```python
from build123d import *

# Parameters (mm, degrees)
ESQUISSE1_W         = 40.75
ESQUISSE1_H         = 20.6
EXTRUSION1_DEPTH    = 9.26
ESQUISSE2_R         = 1.25
EXTRUSION2_DEPTH    = 47.590450738
ESQUISSE4_OUTSIDE_W = 52.068
ESQUISSE4_OUTSIDE_H = 31.918
EXTRUSION5_DEPTH    = 47.590450738
EXTRUSION4_START    = -1.3
EXTRUSION4_DEPTH    = 1.3
EXTRUSION9_DEPTH    = 7.8
EXTRUSION10_REACH   = 48.59
ESQUISSE7_W         = 4
ESQUISSE7_H         = 8.124058542
ESQUISSE8_R         = 2.5
EXTRUSION11_DEPTH   = 4
CONG_1_R            = 5
ESQUISSE9_R         = 2.1
EXTRUSION12_DEPTH   = 1.3


with BuildPart() as part:
    # Esquisse1 → Extrusion1 (new body)
    with BuildSketch(Plane.XY):
        with Locations((-20.375, 10.3)):
            Rectangle(ESQUISSE1_W, ESQUISSE1_H)
    extrude(amount=EXTRUSION1_DEPTH)

    # Esquisse2 → Extrusion2 (cut, through all)
    with BuildSketch(Plane.XY.offset(9.26)):
        with Locations((-38, 17.85)):
            Circle(ESQUISSE2_R)
        with Locations(Location((-38, 2.75, 0), (0, 0, 180))):
            Circle(ESQUISSE2_R)
        with Locations((-2.75, 2.75)):
            Circle(ESQUISSE2_R)
        with Locations(Location((-2.75, 17.85, 0), (0, 0, 180))):
            Circle(ESQUISSE2_R)
    extrude(amount=-EXTRUSION2_DEPTH, mode=Mode.SUBTRACT)

    # Esquisse4 outside → Extrusion5 (cut, through all)
    with BuildSketch(Plane(origin=(0, 0, 0), x_dir=(-1, 0, 0), z_dir=(0, 0, -1))):
        with Locations((20.375, 10.3)):
            Rectangle(ESQUISSE4_OUTSIDE_W, ESQUISSE4_OUTSIDE_H)
        with BuildLine():
            Line((2.75, 20.6), (38, 20.6))
            ThreePointArc((38, 20.6), (39.944543648, 19.794543648), (40.75, 17.85))
            Line((40.75, 17.85), (40.75, 2.75))
            ThreePointArc((40.75, 2.75), (39.944543648, 0.805456352), (38, 0))
            Line((38, 0), (2.75, 0))
            ThreePointArc((2.75, 0), (0.805456352, 0.805456352), (0, 2.75))
            Line((0, 2.75), (0, 17.85))
            ThreePointArc((0, 17.85), (0.805456352, 19.794543648), (2.75, 20.6))
        make_face(mode=Mode.SUBTRACT)
    extrude(amount=-EXTRUSION5_DEPTH, mode=Mode.SUBTRACT)

    # Esquisse3 → Extrusion4 (cut)
    with BuildSketch(Plane.XY.offset(9.26).offset(EXTRUSION4_START)):
        with BuildLine():
            Line((-38, 20.6), (-2.75, 20.6))
            ThreePointArc((-2.75, 20.6), (-0.805456352, 19.794543648), (0, 17.85))
            Line((0, 17.85), (0, 2.75))
            ThreePointArc((0, 2.75), (-0.805456352, 0.805456352), (-2.75, 0))
            Line((-2.75, 0), (-38, 0))
            ThreePointArc((-38, 0), (-39.944543648, 0.805456352), (-40.75, 2.75))
            Line((-40.75, 2.75), (-40.75, 17.85))
            ThreePointArc((-40.75, 17.85), (-39.944543648, 19.794543648), (-38, 20.6))
        make_face()
        with BuildLine():
            Line((-38, 19.6), (-2.75, 19.6))
            ThreePointArc((-2.75, 19.6), (-1.512563133, 19.087436867), (-1, 17.85))
            Line((-1, 17.85), (-1, 2.75))
            ThreePointArc((-1, 2.75), (-1.512563133, 1.512563133), (-2.75, 1))
            Line((-2.75, 1), (-38, 1))
            ThreePointArc((-38, 1), (-39.237436867, 1.512563133), (-39.75, 2.75))
            Line((-39.75, 2.75), (-39.75, 17.85))
            ThreePointArc((-39.75, 17.85), (-39.237436867, 19.087436867), (-38, 19.6))
        make_face(mode=Mode.SUBTRACT)
    extrude(amount=EXTRUSION4_DEPTH, mode=Mode.SUBTRACT)

    # Esquisse6 → Extrusion9 (cut)
    with BuildSketch(Plane.XY.offset(9.26)):
        with BuildLine():
            Line((-36.650926244, 18.8), (-4.099073756, 18.8))
            ThreePointArc((-4.099073756, 18.8), (-3.916726189, 16.683273811), (-1.8, 16.500926244))
            Line((-1.8, 16.500926244), (-1.8, 4.099073756))
            ThreePointArc((-1.8, 4.099073756), (-3.916726189, 3.916726189), (-4.099073756, 1.8))
            Line((-4.099073756, 1.8), (-36.650926244, 1.8))
            ThreePointArc((-36.650926244, 1.8), (-36.833273811, 3.916726189), (-38.95, 4.099073756))
            Line((-38.95, 4.099073756), (-38.95, 16.500926244))
            ThreePointArc((-38.95, 16.500926244), (-36.833273811, 16.683273811), (-36.650926244, 18.8))
        make_face()
    extrude(amount=-EXTRUSION9_DEPTH, mode=Mode.SUBTRACT)

    # Extrusion10: up to this face of the body (flat: up to its plane)
    extrusion10_end = Plane(part.part.faces().sort_by_distance((-38.95, 10.3, 5.36))[0])
    # Esquisse7 → Extrusion10 (cut, up to the picked face)
    with BuildSketch(Plane.ZY.offset(40.75), mode=Mode.PRIVATE) as extrusion10_sk1:
        with Locations((7.26, 10.3)):
            Rectangle(ESQUISSE7_W, ESQUISSE7_H)
    extrusion10_tool1 = split(extrude(extrusion10_sk1.sketch, amount=-EXTRUSION10_REACH, mode=Mode.PRIVATE), bisect_by=extrusion10_end, keep=Keep.BOTH, mode=Mode.PRIVATE)
    add(extrusion10_tool1.solids().sort_by(Axis((-40.75, 10.3, 7.26), (1, 0, 0)))[0], mode=Mode.SUBTRACT)

    # Esquisse8 → Extrusion11 (add)
    # profile 1 of 2: a face of its own
    with BuildSketch(Plane(origin=(0, 0, 0), x_dir=(-1, 0, 0), z_dir=(0, 0, -1))):
        with BuildLine():
            Line((-9, 20.6), (2.75, 20.6))
            ThreePointArc((2.75, 20.6), (0.805456352, 19.794543648), (0, 17.85))
            Line((0, 17.85), (0, 2.75))
            ThreePointArc((0, 2.75), (0.805456352, 0.805456352), (2.75, 0))
            Line((2.75, 0), (-9, 0))
            Line((-9, 0), (-9, 20.6))
        make_face()
        with Locations((-4.5, 15.3)):
            Circle(ESQUISSE8_R, mode=Mode.SUBTRACT)
        with Locations(Location((-4.5, 5.3, 0), (0, 0, 180))):
            Circle(ESQUISSE8_R, mode=Mode.SUBTRACT)
    # profile 2 of 2: a face of its own
    with BuildSketch(Plane(origin=(0, 0, 0), x_dir=(-1, 0, 0), z_dir=(0, 0, -1))):
        with BuildLine():
            Line((49.75, 0), (38, 0))
            ThreePointArc((38, 0), (39.944543648, 0.805456352), (40.75, 2.75))
            Line((40.75, 2.75), (40.75, 17.85))
            ThreePointArc((40.75, 17.85), (39.944543648, 19.794543648), (38, 20.6))
            Line((38, 20.6), (49.75, 20.6))
            Line((49.75, 20.6), (49.75, 0))
        make_face()
        with Locations((45.25, 5.3)):
            Circle(ESQUISSE8_R, mode=Mode.SUBTRACT)
        with Locations(Location((45.25, 15.3, 0), (0, 0, 180))):
            Circle(ESQUISSE8_R, mode=Mode.SUBTRACT)
    extrude(amount=-EXTRUSION11_DEPTH)

    # Congé1
    cong_1_edges = [part.edges().sort_by_distance(p)[0] for p in [
        (9, 0, 2),
        (9, 20.6, 2),
        (-49.75, 20.6, 2),
        (-49.75, 0, 2),
    ]]
    fillet(cong_1_edges, radius=CONG_1_R)

    # Esquisse9 → Extrusion12 (cut)
    with BuildSketch(Plane(origin=(0, 0, 0), x_dir=(-1, 0, 0), z_dir=(0, 0, -1))):
        with Locations((2.75, 17.85)):
            Circle(ESQUISSE9_R)
        with Locations((38, 17.85)):
            Circle(ESQUISSE9_R)
        with Locations((38, 2.75)):
            Circle(ESQUISSE9_R)
        with Locations((2.75, 2.75)):
            Circle(ESQUISSE9_R)
    extrude(amount=-EXTRUSION12_DEPTH, mode=Mode.SUBTRACT)


solid = part.part
```
Could you check a few things on this model? Use its own coordinates, in mm. A direction names the side the tool comes from. Coordinates: 2 decimals unless noted, no trailing zeros. Loops run counter-clockwise (first coordinate to the right, second up) from the corner with the lowest first, then second, coordinate; pieces in that order, holes last. Notation, with made-up numbers: M 79.5,54.5 L 102.5,54.5 A21 cw 102.5,79.5 Z; hole C -22.75,4.5 d2. An arc over 180 degrees is marked long. Put each result on its own line as item: value. Start each with the question number.
(1) I need wall thicknesses on line 1 (Y direction, x = -2.75, z = 0.8); line 2 (Y direction, x = -38, z = 5.75); line 3 (X direction, y = 9.75, z = 4.5). Which ranges of each line are inside material? Lowest first, please. Write a range as from..to.
(2) Will these pins go through, and if not, where does the flat tip stop? P1, Ø3, axis at x = -38, y = 2.75, coming from the +Z side; P2, Ø0.6, axis at y = 13, z = 8.5, coming from the +X side; P3, Ø1.5, axis at x = -2.75, y = 17.85, coming from the -Z side; P4, Ø3, axis at y = 9.5, z = 6.5, coming from the +X side.
(3) For faces 5 (the face through (-4, 2, 1.3)), 6 (the face through (-1, 10, 9)), 7 (the face through (-40.75, 10, 5)), 8 (the face through (-39.92, 19.82, 5.95)), which set-ups out of +Z, -Z, +X, -X, +Y, -Y let a thin tool reach every point of the face, with its end or its side?
(4) Suppose I cut it at B-B on x = -31. Please give me the cut outline in (y, z), then the cut area to 3 significant figures.
(5) Suppose I cut it at A-A on x = -45.5. Please give me the cut outline in (y, z), then the cut area to 3 significant figures.
(6) Thinking about a two-plate mould opening in X: for faces 1 (the face through (9, 10, 2)), 2 (the face through (-40, 10, 5.26)), 3 (the face through (-1.8, 10, 5)), 4 (the face through (-39.75, 4, 9)), which applies, pulls with the +X half, pulls with the -X half, needs draft (parallel to the pull), parting line crosses it, or undercut?
Solutions:
1. line 1: y = 0..0.65, 4.85..15.75, 19.95..20.6
1. line 2: y = 0..1.5, 4..4.4, 16.2..16.6, 19.1..20.6
1. line 3: x = -40.75..-38.95, -1.8..0
2. P1: stops at z = 9.26
2. P2: stops at x = -1
2. P3: passes through
2. P4: stops at x = 0
3. face 5: -Z
3. face 6: +Z, +X, +Y, -Y
3. face 7: +Z, -X, +Y, -Y
3. face 8: +Z, -X, +Y
4. outline: M 0,0 L 20.6,0 L 20.6,7.96 L 19.6,7.96 L 19.6,9.26 L 18.8,9.26 L 18.8,1.46 L 1.8,1.46 L 1.8,9.26 L 1,9.26 L 1,7.96 L 0,7.96 Z
4. area: 55.6 mm2
5. outline: M 0.06,0 L 2.81,0 L 2.81,4 L 0.06,4 Z; M 7.79,0 L 12.81,0 L 12.81,4 L 7.79,4 Z; M 17.79,0 L 20.54,0 L 20.54,4 L 17.79,4 Z
5. area: 42.1 mm2
6. face 1: pulls with the +X half
6. face 2: needs draft
6. face 3: undercut
6. face 4: pulls with the -X half
